```python
from build123d import *
from build123d.topology import SkipClean

# Parameters (mm, degrees)
SKETCH2_W           = 60.23261123
SKETCH2_H           = 92
SKETCH2_W_2         = 59.23261123
SKETCH2_H_2         = 91
BOSS_EXTRUDE1_DEPTH = 3
SKETCH2_2_W         = 60.23261123
SKETCH2_2_H         = 92
BOSS_EXTRUDE2_DEPTH = 1
SKETCH3_W           = 35.019424251
SKETCH3_H           = 3.582680393
BOSS_EXTRUDE3_DEPTH = 1
BOSS_EXTRUDE5_DEPTH = 1
CUT_EXTRUDE2_DEPTH  = 98.380770332


with BuildPart() as part:
    # Sketch2 → Boss-Extrude1 (new body)
    with BuildSketch(Plane(origin=(0, 0, 0), x_dir=(1, 0, 0), z_dir=(0, 1, 0))):
        with Locations((1.344327409, 2.772982692)):
            Rectangle(SKETCH2_W, SKETCH2_H)
        with Locations((1.344327409, 2.772982692)):
            Rectangle(SKETCH2_W_2, SKETCH2_H_2, mode=Mode.SUBTRACT)
    extrude(amount=BOSS_EXTRUDE1_DEPTH)

    # Sketch2<2> → Boss-Extrude2 (add)
    with BuildSketch(Plane(origin=(0, 0, 0), x_dir=(1, 0, 0), z_dir=(0, 1, 0))):
        with Locations((1.344327409, 2.772982692)):
            Rectangle(SKETCH2_2_W, SKETCH2_2_H)
    extrude(amount=-BOSS_EXTRUDE2_DEPTH)

    # Sketch3 → Boss-Extrude3 (add)
    with BuildSketch(Plane.XY.offset(43.227017308)):
        with Locations((1.310252146, 2.334822514)):
            Rectangle(SKETCH3_W, SKETCH3_H)
    extrude(amount=BOSS_EXTRUDE3_DEPTH)

    # Sketch3<5> → Boss-Extrude5 (add)
    with BuildSketch(Plane.XY.offset(43.227017308)):
        with BuildLine():
            Line((29.319964272, 5.407679734), (-26.699459979, 5.407679734))
            ThreePointArc((-26.699459979, 5.407679734), (-28.113673542, 4.821893296), (-28.699459979, 3.407679734))
            Line((-28.699459979, 3.407679734), (-28.699459979, 1.263953606))
            ThreePointArc((-28.699459979, 1.263953606), (-28.113673542, -0.150259957), (-26.699459979, -0.736046394))
            Line((-26.699459979, -0.736046394), (29.319964272, -0.736046394))
            ThreePointArc((29.319964272, -0.736046394), (30.734177835, -0.150259957), (31.319964272, 1.263953606))
            Line((31.319964272, 1.263953606), (31.319964272, 3.407679734))
            ThreePointArc((31.319964272, 3.407679734), (30.734177835, 4.821893296), (29.319964272, 5.407679734))
        make_face()
    extrude(amount=-BOSS_EXTRUDE5_DEPTH)

    # Sketch3<6> → Cut-Extrude2 (cut, through all)
    with SkipClean():  # the faces are left unmerged after this step: merging them gives an invalid solid
        with BuildSketch(Plane.XY.offset(43.227017308)):
            with BuildLine():
                Line((31.460633024, 3), (31.319964272, 3))
                Line((31.319964272, 3), (31.319964272, 1.263953606))
                ThreePointArc((31.319964272, 1.263953606), (30.967290445, 0.129794675), (30.033647793, -0.604376085))
                ThreePointArc((30.033647793, -0.604376085), (29.682828309, -0.702853373), (29.319964272, -0.736046394))
                Line((29.319964272, -0.736046394), (-26.699459979, -0.736046394))
                ThreePointArc((-26.699459979, -0.736046394), (-27.062324016, -0.702853373), (-27.4131435, -0.604376085))
                ThreePointArc((-27.4131435, -0.604376085), (-28.346786152, 0.129794675), (-28.699459979, 1.263953606))
                Line((-28.699459979, 1.263953606), (-28.699459979, 3))
                Line((-28.699459979, 3), (-28.771978206, 3))
                Line((-28.771978206, 3), (-28.771978206, -1))
                Line((-28.771978206, -1), (31.460633024, -1))
                Line((31.460633024, -1), (31.460633024, 3))
            make_face()
        extrude(amount=-CUT_EXTRUDE2_DEPTH, mode=Mode.SUBTRACT)


solid = part.part
```
Can you work these out from the model? Positions are in its coordinate system, mm. A direction names the side the tool comes from. Coordinates: 2 decimals unless noted, no trailing zeros. Order: outer loops, then holes, each group sorted by start corner. A loop starts at its lowest first (then second) coordinate and runs counter-clockwise, first axis right, second up. Notation, with made-up numbers: (42, 9.5) -> (63, 9.5) arc R36 cw to (63, 47.5) -> close; hole circle Ø6 at (-36, -37). An arc over 180 degrees is marked (long way). Write each question's results on one line, items separated by ' | '.
Item 1: If I drill on line 1 along X through (y, z) = (1, 13); line 2 along Z through (x, y) = (17.5, 2.5); line 3 along Z through (x, y) = (-19.5, 1.25), over which ranges is the centre line in solid material (lowest first)?
Results are:
line 1: -28.68 to -28.27, 30.96 to 31.3 | line 2: -48.77 to -48.27, 42.23 to 44.23 | line 3: -48.77 to -48.27, 42.23 to 43.23
Item 2: I want a section at A-A, the plane z = -7. Write out the boundary of the cut face in (x, y), then the cut area to 3 significant figures.
Results are:
outline: (-28.7, 1.26) arc R2 ccw to (-28.27, 0.03) -> (-28.27, 3) -> (-28.7, 3) -> close; (-28.25, 0) arc R2 ccw to (-26.7, -0.74) -> (29.32, -0.74) arc R2 ccw to (30.87, 0) -> close; (30.96, 0.12) arc R2 ccw to (31.32, 1.26) -> (31.32, 3) -> (30.96, 3) -> close | area: 44.8 mm²
Item 3: I want a section at C-C, the plane x = 25.5. Write out the boundary of the cut face in (y, z).
Results are:
outline: (-0.74, -48.77) -> (3, -48.77) -> (3, -48.27) -> (0, -48.27) -> (0, 42.23) -> (5.41, 42.23) -> (5.41, 43.23) -> (-0.74, 43.23) -> close
Item 4: I'm going to push flat-ended pins straight in: pin 1 Ø0.9 at (y, z) = (1, 19.5) entering from +X; pin 2 Ø1.1 at (x, z) = (-6.5, 44) entering from -Y; pin 3 Ø17.5 at (x, z) = (14, -10) entering from +Y. Where does each tip first touch, or does it pass through?
Results are:
pin 1: x = 31.32 | pin 2: y = 0.54 | pin 3: y = 0
Item 5: Which directions (+Z, -Z, +X, -X, +Y, -Y) give clear straight access to the entire face, cutting with the end or side of a thin tool? Please do faces 1 (the face through (1, 3, 42.227)), 2 (the face through (31.32, 2, -2)), 3 (the face through (30.961, 2, -2)).
Results are:
face 1: +Y | face 2: +Z, -Z, +X, +Y, -Y | face 3: +Y, -Y
Item 6: I want a section at B-B, the plane x = -9.5. Write out the boundary of the cut face in (y, z), then the cut area to 3 significant figures.
Results are:
outline: (-0.74, -48.77) -> (3, -48.77) -> (3, -48.27) -> (0, -48.27) -> (0, 42.23) -> (5.41, 42.23) -> (5.41, 43.23) -> (4.13, 43.23) -> (4.13, 44.23) -> (0.54, 44.23) -> (0.54, 43.23) -> (-0.74, 43.23) -> close | area: 78.2 mm²
